from build123d import *

# Parameters (mm, degrees)
BOSS_EXTRUDE1_DEPTH = 20
SKETCH2_R           = 16.25
SKETCH2_R_2         = 2.15
CUT_EXTRUDE1_DEPTH  = 20
SKETCH5_R           = 3.75
CUT_EXTRUDE4_DEPTH  = 4.2
FILLET3_R           = 4
FILLET4_R           = 6.35


with BuildPart() as part:
    # Sketch1 → Boss-Extrude1 (new body)
    with BuildSketch(Plane.XY):
        Polygon((50.8, 25.4), (8.89, 25.4), (8.89, 13.302928249), (-8.89, 13.302928249), (-8.89, 25.4), (-50.8, 25.4), (-50.8, -76.2), (50.8, -76.2), align=None)
    extrude(amount=BOSS_EXTRUDE1_DEPTH)

    # Sketch2 → Cut-Extrude1 (cut)
    with BuildSketch(Plane.XY.offset(20)):
        Circle(SKETCH2_R)
        with Locations((-15.5, -15.5)):
            Circle(SKETCH2_R_2)
        with Locations((-15.5, 15.5)):
            Circle(SKETCH2_R_2)
        with Locations((15.5, -15.5)):
            Circle(SKETCH2_R_2)
        with Locations((15.5, 15.5)):
            Circle(SKETCH2_R_2)
    extrude(amount=-CUT_EXTRUDE1_DEPTH, mode=Mode.SUBTRACT)

    # Sketch5 → Cut-Extrude4 (cut)
    with BuildSketch(Plane.XY.offset(20)):
        with Locations((-15.5, 15.5)):
            Circle(SKETCH5_R)
        with Locations((15.5, 15.5)):
            Circle(SKETCH5_R)
        with Locations((15.5, -15.5)):
            Circle(SKETCH5_R)
        with Locations((-15.5, -15.5)):
            Circle(SKETCH5_R)
    extrude(amount=-CUT_EXTRUDE4_DEPTH, mode=Mode.SUBTRACT)

    # Fillet3
    fillet3_edges = [part.edges().sort_by_distance(p)[0] for p in [
        (8.89, 13.602587989, 10),
        (-8.89, 13.602587989, 10),
    ]]
    fillet(fillet3_edges, radius=FILLET3_R)

    # Fillet4
    fillet4_edges = [part.edges().sort_by_distance(p)[0] for p in [
        (-50.8, 25.4, 10),
        (-8.89, 25.4, 10),
        (8.89, 25.4, 10),
        (50.8, 25.4, 10),
    ]]
    fillet(fillet4_edges, radius=FILLET4_R)


solid = part.part
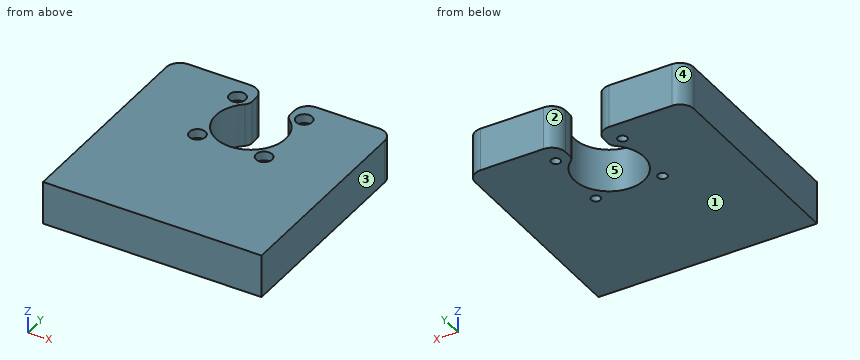
Verification items for the finished model (mm, model axes). Face numbers are marked on the shaded views. A direction names the side the tool comes from. Give positions to 0.01 mm unless a question says otherwise; leave off trailing zeros. Order: outer loops, then holes, each group sorted by start corner. A loop starts at its lowest first (then second) coordinate and runs counter-clockwise, first axis right, second up. Notation, with made-up numbers: M 40,70 L 90,70 A24 ccw 90,100 Z; hole C 72.25,-19.5 d4. An arc over 180 degrees is marked long. Use one line per item in the form item = value. Start each with the question number.
Q1. Section check A-A (y = 0). Enter the section's corners in (x, z).
Q2. Access from +Z, -Z, +X, -X, +Y, -Y to the whole of each face (thin tool, end or side, straight path). Record for the marked faces 1 and 2.
Q3. Go/stop test with a flat-tipped pin: pin 1 Ø4 at (x, y) = (14.5, -15) entering from +Z. Record where the tip stops, or that it passes through.
Q4. Scan lines: line 1 along X through (y, z) = (0, 4.5); line 2 along X through (y, z) = (-14, 5); line 3 along Y through (x, z) = (-17, 5.25). Record each from-to range of solid material in increasing order. Write a range as [from, to].
Q5. Mould release check, pull along Y, two halves, no side actions. Record for the marked faces 3, 4 and 5: +Y half, -Y half, draft (parallel to the pull), parting line (faces both ways), or undercut.
Q6. Section check B-B (z = 18). Enter the section's corners in (x, y), then the cut area to 3 significant figures.
Q7. Section check D-D (x = 7). Enter the section's corners in (y, z) (3 decimals).
Q8. Section check C-C (x = -6). Enter the section's corners in (y, z), then the cut area to 3 significant figures.
Evaluation:
q1.outline = M -50.8,0 L -16.25,0 L -16.25,20 L -50.8,20 Z; M 16.25,0 L 50.8,0 L 50.8,20 L 16.25,20 Z
q2.face_1 = -Z, +X, -X, +Y, -Y
q2.face_2 = +Z, -Z, +Y
q3.pin_1 = 15.8
q4.line_1 = [-50.8, -16.25], [16.25, 50.8]
q4.line_2 = [-50.8, -17.04], [-13.96, -8.25], [8.25, 13.96], [17.04, 50.8]
q4.line_3 = [-76.2, -17.04], [-13.96, 13.96], [17.04, 25.4]
q5.face_3 = draft
q5.face_4 = +Y half
q5.face_5 = undercut
q6.outline = M -50.8,-76.2 L 50.8,-76.2 L 50.8,19.05 A6.35 ccw 44.45,25.4 L 15.24,25.4 A6.35 ccw 8.89,19.05 L 8.89,15.62 A4 ccw 10.34,12.53 A16.25 cw long -10.34,12.53 A4 ccw -8.89,15.62 L -8.89,19.05 A6.35 ccw -15.24,25.4 L -44.45,25.4 A6.35 ccw -50.8,19.05 Z; hole C -15.5,-15.5 d7.5; hole C -15.5,15.5 d7.5; hole C 15.5,-15.5 d7.5; hole C 15.5,15.5 d7.5
q6.area = 9,100 mm2
q7.outline = M -76.2,0 L -14.665,0 L -14.665,20 L -76.2,20 Z
q8.outline = M -76.2,0 L -15.1,0 L -15.1,20 L -76.2,20 Z
q8.area = 1,220 mm2
